The listing builds one solid part. Answer for the finished solid, in the listing's coordinates (mm). A direction names the side the tool comes from. Round coordinates to 2 decimals unless told otherwise and drop trailing zeros. Order: outer loops, then holes, each group sorted by start corner. A loop starts at its lowest first (then second) coordinate and runs counter-clockwise, first axis right, second up. Notation, with made-up numbers: M 52,-0.75 L 62,-0.75 A21 ccw 62,5.25 Z; hole C -10.75,6.5 d6. An arc over 180 degrees is marked long. Put each result on its own line as item: value. Start each with the question number.
1. This flat-tipped pin is pushed along its axis until it touches: pin 1 Ø4 at (y, z) = (9.76, 63.65) entering from -X. Where does it stop, or does it pass through?
2. Consider line 1 (Y direction, x = 22, z = 49). Determine where the line is inside the solid, lowest interval first.
3. Which of the six approach directions +Z, -Z, +X, -X, +Y, -Y give full straight-line access (tool end or side, diameter ignored) to faces 1 (the face through (0.3, 44.07, 61.42)), 2 (the face through (0, 35, 35)), 3 (the face through (69.4, 35, 35))?
4. The part is cut by section D-D (z = 30). Give the vertices of the cut face in (x, y), then the cut area to 3 significant figures.
5. The part is cut by section B-B (z = 63.65). Give the vertices of the cut face in (x, y).
6. The part is cut by section A-A (x = 60). Give the vertices of the cut face in (y, z).
7. The mould has two halves that part along X. Classify faces 4 (the face through (35, 69.4, 35)), 5 (the face through (70, 35, 35)), 6 (the face through (35, 0, 35)): +X half, -X half, draft (parallel to the pull), parting line (faces both ways), or undercut.
from build123d import *

# Parameters (mm, degrees)
CROQUIS1_W                        = 70
CROQUIS1_H                        = 70
SALIENTE_EXTRUIR1_DEPTH           = 70
VACIADO1_T                        = -0.6
TALADRO_DE_MARGEN_PARA_M41_REACH  = 173.7
TALADRO_DE_MARGEN_PARA_M41_BORE_R = 2.25


with BuildPart() as part:
    # Croquis1 → Saliente-Extruir1 (new body)
    with BuildSketch(Plane.XY):
        with Locations((35, 35)):
            Rectangle(CROQUIS1_W, CROQUIS1_H)
    extrude(amount=SALIENTE_EXTRUIR1_DEPTH)

    # Vaciado1
    vaciado1_openings = [part.faces().sort_by_distance(p)[0] for p in [
        (35, 35, 70),
        (35, 35, 0),
    ]]
    offset(amount=VACIADO1_T, openings=vaciado1_openings, kind=Kind.INTERSECTION)

    # Taladro de margen para M41 bore → Taladro de margen para M41 (cut, up to next)
    with BuildSketch(Plane(origin=(-1, -81.2, 39.730415546), x_dir=(0, 1, 0), z_dir=(-1, 0, 0)), mode=Mode.PRIVATE) as taladro_de_margen_para_m41_sk1:
        with Locations((90.9625, -23.919584454)):
            Circle(TALADRO_DE_MARGEN_PARA_M41_BORE_R)
    taladro_de_margen_para_m41_tool1 = extrude(taladro_de_margen_para_m41_sk1.sketch, amount=-TALADRO_DE_MARGEN_PARA_M41_REACH, mode=Mode.PRIVATE) & part.part
    # Taladro de margen para M41 bore → Taladro de margen para M41 (cut, up to next)
    with BuildSketch(Plane(origin=(-1, -81.2, 39.730415546), x_dir=(0, 1, 0), z_dir=(-1, 0, 0)), mode=Mode.PRIVATE) as taladro_de_margen_para_m41_sk2:
        with Locations((106.8375, -23.919584454)):
            Circle(TALADRO_DE_MARGEN_PARA_M41_BORE_R)
    taladro_de_margen_para_m41_tool2 = extrude(taladro_de_margen_para_m41_sk2.sketch, amount=-TALADRO_DE_MARGEN_PARA_M41_REACH, mode=Mode.PRIVATE) & part.part
    # Taladro de margen para M41 bore → Taladro de margen para M41 (cut, up to next)
    with BuildSketch(Plane(origin=(-1, -81.2, 39.730415546), x_dir=(0, 1, 0), z_dir=(-1, 0, 0)), mode=Mode.PRIVATE) as taladro_de_margen_para_m41_sk3:
        with Locations((125.5625, -23.919584454)):
            Circle(TALADRO_DE_MARGEN_PARA_M41_BORE_R)
    taladro_de_margen_para_m41_tool3 = extrude(taladro_de_margen_para_m41_sk3.sketch, amount=-TALADRO_DE_MARGEN_PARA_M41_REACH, mode=Mode.PRIVATE) & part.part
    # Taladro de margen para M41 bore → Taladro de margen para M41 (cut, up to next)
    with BuildSketch(Plane(origin=(-1, -81.2, 39.730415546), x_dir=(0, 1, 0), z_dir=(-1, 0, 0)), mode=Mode.PRIVATE) as taladro_de_margen_para_m41_sk4:
        with Locations((141.4375, -23.919584454)):
            Circle(TALADRO_DE_MARGEN_PARA_M41_BORE_R)
    taladro_de_margen_para_m41_tool4 = extrude(taladro_de_margen_para_m41_sk4.sketch, amount=-TALADRO_DE_MARGEN_PARA_M41_REACH, mode=Mode.PRIVATE) & part.part
    add(taladro_de_margen_para_m41_tool1.solids().sort_by_distance((-1, 9.7625, 63.65))[0], mode=Mode.SUBTRACT)
    add(taladro_de_margen_para_m41_tool2.solids().sort_by_distance((-1, 25.6375, 63.65))[0], mode=Mode.SUBTRACT)
    add(taladro_de_margen_para_m41_tool3.solids().sort_by_distance((-1, 44.3625, 63.65))[0], mode=Mode.SUBTRACT)
    add(taladro_de_margen_para_m41_tool4.solids().sort_by_distance((-1, 60.2375, 63.65))[0], mode=Mode.SUBTRACT)


solid = part.part
Resolved:
1. pin 1: x = 69.4
2. line 1: 0 to 0.6, 69.4 to 70
3. face 1: -X
3. face 2: +Z, -Z, -X, +Y, -Y
3. face 3: +Z, -Z
4. outline: M 0,0 L 70,0 L 70,70 L 0,70 Z; hole M 0.6,0.6 L 69.4,0.6 L 69.4,69.4 L 0.6,69.4 Z
4. area: 167 mm2
5. outline: M 0,0 L 70,0 L 70,70 L 0,70 L 0,62.49 L 0.6,62.49 L 0.6,69.4 L 69.4,69.4 L 69.4,0.6 L 0.6,0.6 L 0.6,7.51 L 0,7.51 Z; M 0,12.01 L 0.6,12.01 L 0.6,23.39 L 0,23.39 Z; M 0,27.89 L 0.6,27.89 L 0.6,42.11 L 0,42.11 Z; M 0,46.61 L 0.6,46.61 L 0.6,57.99 L 0,57.99 Z
6. outline: M 0,0 L 0.6,0 L 0.6,70 L 0,70 Z; M 69.4,0 L 70,0 L 70,70 L 69.4,70 Z
7. face 4: undercut
7. face 5: +X half
7. face 6: draft
